```python
from build123d import *

# Parameters (mm, degrees)
SKIZZE1_W                       = 9.5
SKIZZE1_H                       = 11.093
SKIZZE1_W_2                     = 8.7
SKIZZE1_H_2                     = 4.7
SKIZZE1_H_3                     = 5.193
AUFSATZ_LINEAR_AUSTRAGEN1_DEPTH = 22
AUFSATZ_LINEAR_AUSTRAGEN2_DEPTH = 2.3
SCHNITT_LINEAR_AUSTRAGEN1_DEPTH = 13.7
SKIZZE4_W                       = 13.3
SKIZZE4_H                       = 5.193
SCHNITT_LINEAR_AUSTRAGEN2_DEPTH = 0.4
SKIZZE5_W                       = 14.1
SKIZZE5_H                       = 0.4
AUFSATZ_LINEAR_AUSTRAGEN3_DEPTH = 20
AUFSATZ_LINEAR_AUSTRAGEN4_DEPTH = 0.2


with BuildPart() as part:
    # Skizze1 → Aufsatz-Linear austragen1 (new body)
    with BuildSketch(Plane(origin=(0, 0, 0), x_dir=(1, 0, 0), z_dir=(0, 1, 0))):
        with Locations((4.75, 5.5465)):
            Rectangle(SKIZZE1_W, SKIZZE1_H)
        with Locations((4.75, 2.75)):
            Rectangle(SKIZZE1_W_2, SKIZZE1_H_2, mode=Mode.SUBTRACT)
        with Locations((4.75, 8.0965)):
            Rectangle(SKIZZE1_W_2, SKIZZE1_H_3, mode=Mode.SUBTRACT)
    extrude(amount=AUFSATZ_LINEAR_AUSTRAGEN1_DEPTH)

    # Skizze2 → Aufsatz-Linear austragen2 (add)
    with BuildSketch(Plane.ZY):
        Polygon((-11.093, 0), (-11.093, 3.67), (-8.093, 13.8), (-5.093, 3.67), (-5.093, 0), align=None)
    aufsatz_linear_austragen2 = extrude(amount=AUFSATZ_LINEAR_AUSTRAGEN2_DEPTH)

    # Spiegeln1: Aufsatz-Linear austragen2 across plane
    add(aufsatz_linear_austragen2.mirror(Plane(origin=(4.75, 0, 0), x_dir=(0, 0, 1), z_dir=(1, 0, 0))))

    # Skizze3 → Schnitt-Linear austragen1 (cut)
    with BuildSketch(Plane.ZY.offset(2.3)):
        Polygon((-10.693, 0.4), (-5.493, 0.4), (-5.493, 3.612014671), (-8.093, 12.391348004), (-10.693, 3.612014671), align=None)
    extrude(amount=-SCHNITT_LINEAR_AUSTRAGEN1_DEPTH, mode=Mode.SUBTRACT)

    # Skizze4 → Schnitt-Linear austragen2 (cut)
    with BuildSketch(Plane.XZ):
        with Locations((4.75, -8.0965)):
            Rectangle(SKIZZE4_W, SKIZZE4_H)
    extrude(amount=-SCHNITT_LINEAR_AUSTRAGEN2_DEPTH, mode=Mode.SUBTRACT)

    # Skizze5 → Aufsatz-Linear austragen3 (add)
    with BuildSketch(Plane.XZ):
        with Locations((4.75, -10.893)):
            Rectangle(SKIZZE5_W, SKIZZE5_H)
    extrude(amount=AUFSATZ_LINEAR_AUSTRAGEN3_DEPTH)

    # Skizze6 → Aufsatz-Linear austragen4 (add)
    with BuildSketch(Plane(origin=(0, 0, -11.093), x_dir=(-1, 0, 0), z_dir=(0, 0, -1))):
        Polygon((0, 3.67), (2.3, 3.67), (2.3, -20), (-11.8, -20), (-11.8, 3.67), (-9.5, 3.67), (-9.5, 22), (0, 22), align=None)
    extrude(amount=AUFSATZ_LINEAR_AUSTRAGEN4_DEPTH)


solid = part.part
```
Design review of the part built by this model. Coordinates are the model's own, in mm. A direction names the side the tool comes from. Coordinates: 2 decimals unless noted, no trailing zeros. Loops run counter-clockwise (first coordinate to the right, second up) from the corner with the lowest first, then second, coordinate; pieces in that order, holes last. Notation, with made-up numbers: (23.5, 4) -> (37.5, 4) arc R15 ccw to (37.5, 18) -> close; hole circle Ø2 at (73.5, 6.5). An arc over 180 degrees is marked (long way). Answer as a JSON object with one key per item and string values.
Q1. Take a section at C-C on y = 19.5. Give the boundary of the cut face in (x, z).
Answer block:
{"outline": "(0, -11.29) -> (9.5, -11.29) -> (9.5, 0) -> (0, 0) -> close; hole (0.4, -10.69) -> (9.1, -10.69) -> (9.1, -5.5) -> (0.4, -5.5) -> close; hole (0.4, -5.1) -> (9.1, -5.1) -> (9.1, -0.4) -> (0.4, -0.4) -> close"}
Q2. Take a section at A-A on z = -1.75. Give the boundary of the cut face in (x, y).
Answer block:
{"outline": "(0, 0) -> (0.4, 0) -> (0.4, 22) -> (0, 22) -> close; (9.1, 0) -> (9.5, 0) -> (9.5, 22) -> (9.1, 22) -> close"}
Q3. The part is to be moulded in two halves that separate along Z. For faces 1 (the flat face through (9.5, 13, -4)), 2 (the flat face through (5, 11, 0)), 3 (the flat face through (-1.134, 8.664, -9.614)), 4 (the flat face through (5, 11, -5.1)), say which applies: +Z half, -Z half, draft (parallel to the pull), parting line (faces both ways), or undercut.
Answer block:
{"face 1": "draft", "face 2": "+Z half", "face 3": "-Z half", "face 4": "undercut"}
Q4. Clearance check with flat-ended pins moving along their axes: pin 1 Ø3.5 at (y, z) = (15, -4.5) entering from -X; pin 2 Ø2.5 at (y, z) = (16, -3) entering from +X; pin 3 Ø2.5 at (x, y) = (-1.5, 1.5) entering from +Z; pin 4 Ø1.6 at (x, z) = (2.5, -7) entering from +Y. State where each tip first meets the part, or that it passes through.
Answer block:
{"pin 1": "stops at x = 0", "pin 2": "stops at x = 9.5", "pin 3": "stops at z = -5.09", "pin 4": "passes through"}
Q5. To check wall thickness, follow L1, parallel to Z at x = 6.75, y = 13; L2, parallel to X at y = 18.5, z = -3.75; L3, parallel to Z at x = 9.5, y = -1. State the ranges of each line that lie inside material, in increasing order.
Answer block:
{"L1": "z = -11.29 to -10.69, -5.5 to -5.1, -0.4 to 0", "L2": "x = 0 to 0.4, 9.1 to 9.5", "L3": "z = -11.29 to -10.69"}
Q6. Take a section at B-B on x = 6.5. Give the number of separate pieces and of enclosed holes in the cut face, plus the area to 3 significant figures.
Answer block:
{"separate pieces": "3", "enclosed holes": "0", "area": "42.8 mm^2"}
Q7. Tool access review of faces 5 (the flat face through (-1.134, 8.806, -6.614)), 6 (the flat face through (10.634, 8.664, -9.614)), 7 (the flat face through (0.4, 11, -3)): name each direction out of +Z, -Z, +X, -X, +Y, -Y from which nothing blocks a thin tool from reaching the whole face with its end or side.
Answer block:
{"face 5": "+Z, -X, +Y", "face 6": "-Z, +X, +Y", "face 7": "+Y, -Y"}
